Here's how the part is built. I have some questions about the finished solid (model axes, mm). Give positions to 0.01 mm unless a question says otherwise; leave off trailing zeros. Loops run counter-clockwise (first coordinate to the right, second up) from the corner with the lowest first, then second, coordinate; pieces in that order, holes last.
Q1. I need wall thicknesses on line 1 (X direction, y = 1.05, z = -23.5); line 2 (Z direction, x = 3.25, y = 0.55) (3 decimals); line 3 (X direction, y = 0.5, z = -22.5). Which ranges of each line are inside material? Lowest first, please.
Q2. Will these pins go through, and if not, where does the flat tip stop? P1, Ø6, axis at x = 12, z = -22, coming from the -Y side; P2, Ø0.5, axis at x = 1, y = 1, coming from the -Z side (3 decimals); P3, Ø0.9, axis at x = 24.5, y = 0.5, coming from the -Z side; P4, Ø0.5, axis at y = 1, z = -26.5, coming from the +X side.
Q3. If we section it at B-B (x = 2.54): Please give me the cut outline in (y, z) (3 decimals).
Q4. If we section it at A-A (z = -27): Please give me the cut outline in (x, y).
Autodesk Inventor part; units mm, degrees
ref_plane "YZ Plane" through (0, 0, 0) normal (1, 0, 0) x (0, 1, 0)
ref_plane "XZ Plane" through (0, 0, 0) normal (0, 1, 0) x (-1, 0, 0)
ref_plane "XY Plane" through (0, 0, 0) normal (0, 0, 1) x (1, 0, 0)
sketch "Sketch1" plane through (0, 0, 0) normal (0, 1, 0) x (-1, 0, 0)
  line L0 (0, 0) -> (-28.321, 0) construction
  line L1 (-28.321, 0) -> (-28.321, -22.225)
  line L2 (-28.321, -22.225) -> (0, -22.225) construction
  line L3 (0, -22.225) -> (0, 0)
  line L4 (-1.778, 0) -> (-3.048, 0) construction
  line L5 (-3.048, 0) -> (-3.048, -0.635)
  line L6 (-2.413, -1.27) -> (-2.413, -1.27)
  line L7 (-1.778, -0.635) -> (-1.778, 0)
  arc A0 (-2.413, -1.27) -> (-1.778, -0.635) centre (-2.413, -0.635) ccw
  arc A1 (-3.048, -0.635) -> (-2.413, -1.27) centre (-2.413, -0.635) ccw
  line L8 (0, 0) -> (-1.778, 0)
  line L9 (0, -11.1125) -> (-6.6148, -11.1125) construction
  line L10 (-14.1605, -22.225) -> (-14.1605, -12.0846) construction
  line L11 (-25.273, 0) -> (-26.543, 0) construction
  line L12 (-26.543, 0) -> (-26.543, -0.635)
  line L13 (-25.908, -1.27) -> (-25.908, -1.27)
  line L14 (-25.273, -0.635) -> (-25.273, 0)
  arc A2 (-25.908, -1.27) -> (-25.273, -0.635) centre (-25.908, -0.635) ccw
  arc A3 (-26.543, -0.635) -> (-25.908, -1.27) centre (-25.908, -0.635) ccw
  line L15 (-26.543, 0) -> (-28.321, 0)
  line L16 (-25.273, 0) -> (-3.048, 0)
  line L17 (-25.146, -22.225) -> (-26.416, -22.225) construction
  line L18 (-26.416, -22.225) -> (-26.416, -21.59)
  line L19 (-25.781, -20.955) -> (-25.781, -20.955)
  line L20 (-25.146, -21.59) -> (-25.146, -22.225)
  line L21 (-1.905, -22.225) -> (-3.175, -22.225) construction
  line L22 (-3.175, -22.225) -> (-3.175, -21.59)
  line L23 (-2.54, -20.955) -> (-2.54, -20.955)
  line L24 (-1.905, -21.59) -> (-1.905, -22.225)
  line L25 (0, -22.225) -> (-1.905, -22.225)
  arc A4 (-1.905, -21.59) -> (-2.54, -20.955) centre (-2.54, -21.59) ccw
  arc A5 (-2.54, -20.955) -> (-3.175, -21.59) centre (-2.54, -21.59) ccw
  arc A6 (-25.146, -21.59) -> (-25.781, -20.955) centre (-25.781, -21.59) ccw
  arc A7 (-25.781, -20.955) -> (-26.416, -21.59) centre (-25.781, -21.59) ccw
  line L26 (-26.416, -22.225) -> (-28.321, -22.225)
  line L27 (-4.0005, -22.225) -> (-24.3205, -22.225) construction
  line L28 (-24.3205, -22.225) -> (-24.3205, -30.099)
  line L29 (-23.8125, -30.607) -> (-4.5085, -30.607) construction
  line L30 (-4.0005, -30.099) -> (-4.0005, -22.225)
  line L31 (-4.5085, -30.607) -> (-4.0005, -30.099)
  line L32 (-23.8125, -30.607) -> (-24.3205, -30.099)
  line L33 (-11.303, -30.607) -> (-13.208, -30.607) construction
  line L34 (-13.208, -30.099) -> (-13.208, -23.1775)
  line L35 (-12.2555, -22.225) -> (-12.2555, -22.225)
  line L36 (-11.303, -23.1775) -> (-11.303, -30.099)
  arc A8 (-12.2555, -22.225) -> (-13.208, -23.1775) centre (-12.2555, -23.1775) ccw
  arc A9 (-11.303, -23.1775) -> (-12.2555, -22.225) centre (-12.2555, -23.1775) ccw
  line L37 (-13.716, -30.607) -> (-23.8125, -30.607)
  line L38 (-10.795, -30.607) -> (-4.5085, -30.607)
  line L39 (-4.0005, -22.225) -> (-3.175, -22.225)
  line L40 (-25.146, -22.225) -> (-24.3205, -22.225)
  line L41 (-10.795, -30.607) -> (-11.303, -30.099)
  line L42 (-13.208, -30.099) -> (-13.716, -30.607)
  point P0 (-2.413, 0)
  point P1 (-26.543, -1.27)
  point P2 (-25.273, -1.27)
  point P3 (-25.908, 0)
  point P4 (-2.54, -22.225)
  point P5 (-25.781, -22.225)
  point P6 (-24.3205, -30.607)
  point P7 (-4.0005, -30.607)
  point P8 (-13.208, -22.225)
  dimension "d0" = 22.225
  dimension "d1" = 28.321
  dimension "d2" = 1.27
  dimension "d3" = 2.413
  dimension "d4" = 1.27
  dimension "d5" = 0.635
  dimension "d6" = 1.27
  dimension "d7" = 1.27
  dimension "d8" = 2.413
  dimension "d9" = 0.635
  dimension "d12" = 1.27
  dimension "d13" = 1.27
  dimension "d14" = 1.27
  dimension "d15" = 1.27
  dimension "d16" = 2.54
  dimension "d17" = 0.635
  dimension "d18" = 2.54
  dimension "d19" = 0.635
  dimension "d20" = 20.32
  dimension "d21" = 0.508
  dimension "d22" = 0.508
  dimension "d23" = 0.508
  dimension "d24" = 0.508
  dimension "d25" = 8.382
  dimension "d26" = 1.905
  dimension "d27" = 0.9525
  dimension "d28" = 8.255
  dimension "d29" = 0.508
  dimension "d30" = 0.508
  dimension "d31" = 0.508
  dimension "d32" = 0.508
  dimension "d40" = 23.495
extrude "Extrusion1" add sketch "Sketch1" along normal blind 1.64
sketch "Sketch2" plane through (0, 1.64, 0) normal (0, 1, 0) x (1, 0, 0)
  line L0 (6, -1) -> (22.321, -1)
  line L1 (22.321, -1) -> (22.321, 6)
  line L2 (22.321, 6) -> (6, 6)
  line L3 (6, 6) -> (6, -1)
  line L4 (0, 22.225) -> (0, 0)
  line L5 (28.321, 0) -> (28.321, 22.225)
  line L6 (3.048, 0) -> (25.273, 0)
  dimension "d35" = 7
  dimension "d36" = 6
  dimension "d37" = 6
  dimension "d38" = 1
equation "\"d30\" = d29"
equation "\"d31\" = d29"
equation "\"d32\" = d31"
properties part number "HDMI Plugin Module"
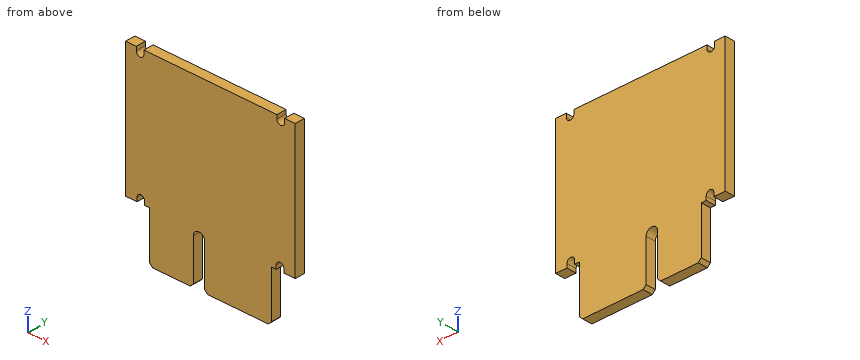
Check sheet entries:
1. line 1: x = 4 to 11.3, 13.21 to 24.32
1. line 2: z = -22.225 to 0
1. line 3: x = 4 to 11.59, 12.93 to 24.32
2. P1: stops at y = 0
2. P2: stops at z = -22.225
2. P3: stops at z = -30.37
2. P4: stops at x = 24.32
3. outline: (0, -20.955) - (1.64, -20.955) - (1.64, -1.257) - (0, -1.257) - close
4. outline: (4, 0) - (11.3, 0) - (11.3, 1.64) - (4, 1.64) - close; (13.21, 0) - (24.32, 0) - (24.32, 1.64) - (13.21, 1.64) - close
